Read the model definition and answer for the solid it produces. Units are mm, in the model's axes. A direction names the side the tool comes from. Round coordinates to 2 decimals unless told otherwise and drop trailing zeros. Write each loop counter-clockwise with the first axis right and the second up, starting at its lowest first coordinate (ties: lowest second). Pieces come first, ordered by that corner, then holes.
from build123d import *

# Parameters (mm, degrees)
SKETCH_1_W                   = 85.6
SKETCH_1_H                   = 90
EXTRUDE_1_DEPTH              = 6
SKETCH_2_W                   = 85.6
SKETCH_2_H                   = 17.95
EXTRUDE_2_DEPTH              = 0.2
SKETCH_3_W                   = 40
SKETCH_3_H                   = 30
CUT_EXTRUDE_1_DEPTH          = 7
HOLE_WIZARD_M4_1_D           = 4.5
HOLE_WIZARD_M4_1_CBORE_D     = 8
HOLE_WIZARD_M4_1_CBORE_DEPTH = 4.4


with BuildPart() as part:
    # 草图1 → 凸台-拉伸1 (new body)
    with BuildSketch(Plane.XY):
        with Locations((42.8, 45)):
            Rectangle(SKETCH_1_W, SKETCH_1_H)
    extrude(amount=EXTRUDE_1_DEPTH)

    # 草图2 → 凸台-拉伸2 (add)
    with BuildSketch(Plane.XY.offset(6)):
        with Locations((42.8, 81.025)):
            Rectangle(SKETCH_2_W, SKETCH_2_H)
        with Locations((42.8, 8.975)):
            Rectangle(SKETCH_2_W, SKETCH_2_H)
    extrude(amount=EXTRUDE_2_DEPTH)

    # 草图3 → 切除-拉伸1 (cut, through all)
    with BuildSketch(Plane.XY.offset(6)):
        with Locations((20, 45)):
            Rectangle(SKETCH_3_W, SKETCH_3_H)
    extrude(amount=-CUT_EXTRUDE_1_DEPTH, mode=Mode.SUBTRACT)

    # M4 六角凹头螺钉的柱形沉头孔1 (through all)
    with Locations(Plane.XY.offset(6.2)):
        with Locations((77.8, 80), (7.8, 80), (7.8, 10), (77.8, 10)):
            CounterBoreHole(HOLE_WIZARD_M4_1_D / 2, HOLE_WIZARD_M4_1_CBORE_D / 2, HOLE_WIZARD_M4_1_CBORE_DEPTH)


solid = part.part
Q1. Section B-B (x = 7.8) is taken. Determine the outline of the cut face in (y, z), then the cut area to 3 significant figures.
Verdict:
outline: (0, 0) - (7.75, 0) - (7.75, 1.8) - (6, 1.8) - (6, 6.2) - (0, 6.2) - close; (12.25, 0) - (30, 0) - (30, 6) - (17.95, 6) - (17.95, 6.2) - (14, 6.2) - (14, 1.8) - (12.25, 1.8) - close; (60, 0) - (77.75, 0) - (77.75, 1.8) - (76, 1.8) - (76, 6.2) - (72.05, 6.2) - (72.05, 6) - (60, 6) - close; (82.25, 0) - (90, 0) - (90, 6.2) - (84, 6.2) - (84, 1.8) - (82.25, 1.8) - close
area: 281 mm2
Q2. Which of the six approach directions +Z, -Z, +X, -X, +Y, -Y give full straight-line access (tool end or side, diameter ignored) to faces 5 (the flat face through (20, 30, 3)), 6 (the flat face through (0, 15, 3)), 7 (the flat face through (10, 8, 1.8))?
Verdict:
face 5: +Z, -Z, -X
face 6: +Z, -Z, -X, +Y, -Y
face 7: +Z
Q3. Section A-A (x = 38) is taken. Determine the outline of the cut face in (y, z), then the cut area to 3 significant figures.
Verdict:
outline: (0, 0) - (30, 0) - (30, 6) - (17.95, 6) - (17.95, 6.2) - (0, 6.2) - close; (60, 0) - (90, 0) - (90, 6.2) - (72.05, 6.2) - (72.05, 6) - (60, 6) - close
area: 367 mm2
Q4. Section D-D (z = 4.75) is taken. Determine the outline of the cut face in (x, y), then the cut area to 3 significant figures.
Verdict:
outline: (0, 0) - (85.6, 0) - (85.6, 90) - (0, 90) - (0, 60) - (40, 60) - (40, 30) - (0, 30) - close; hole circle Ø8 at (7.8, 10); hole circle Ø8 at (7.8, 80); hole circle Ø8 at (77.8, 10); hole circle Ø8 at (77.8, 80)
area: 6,300 mm2
Q5. Section C-C (y = 10) is taken. Determine the outline of the cut face in (x, z).
Verdict:
outline: (0, 0) - (5.55, 0) - (5.55, 1.8) - (3.8, 1.8) - (3.8, 6.2) - (0, 6.2) - close; (10.05, 0) - (75.55, 0) - (75.55, 1.8) - (73.8, 1.8) - (73.8, 6.2) - (11.8, 6.2) - (11.8, 1.8) - (10.05, 1.8) - close; (80.05, 0) - (85.6, 0) - (85.6, 6.2) - (81.8, 6.2) - (81.8, 1.8) - (80.05, 1.8) - close
Q6. Straight lines are drawn through the part: probe 1 along Y at (x, z) = (7.8, 1.25); probe 2 along Y at (x, z) = (77.8, 4.55); probe 3 along Y at (x, z) = (39, 5.25). For each, find the intervals that lie inside material, in ascending order.
Verdict:
probe 1: y = 0 to 7.75, 12.25 to 30, 60 to 77.75, 82.25 to 90
probe 2: y = 0 to 6, 14 to 76, 84 to 90
probe 3: y = 0 to 30, 60 to 90
Q7. Flat-ended cylindrical pins translate along their axes: pin 1 Ø1.5 at (y, z) = (52.5, 5) entering from -X; pin 2 Ø1.5 at (x, y) = (24.5, 75.5) entering from -Z; pin 3 Ø2.5 at (x, y) = (78.5, 78.5) entering from +Z. Find the tip coordinate at first contact, or state that the pin passes through.
Verdict:
pin 1: stops at x = 40
pin 2: stops at z = 0
pin 3: stops at z = 1.8
Q8. Determine the mould class of faces 1 (the cylindrical face through (76.933, 76.095, 4.031)), 2 (the flat face through (52, 45, 6)), 3 (the cylindrical face through (8.288, 77.804, 0.887)), 4 (the flat face through (0, 75, 3)) for opening direction X: pulls with the +X half, pulls with the -X half, needs draft (parallel to the pull), parting line crosses it, or undercut.
Verdict:
face 1: undercut
face 2: needs draft
face 3: undercut
face 4: pulls with the -X half
